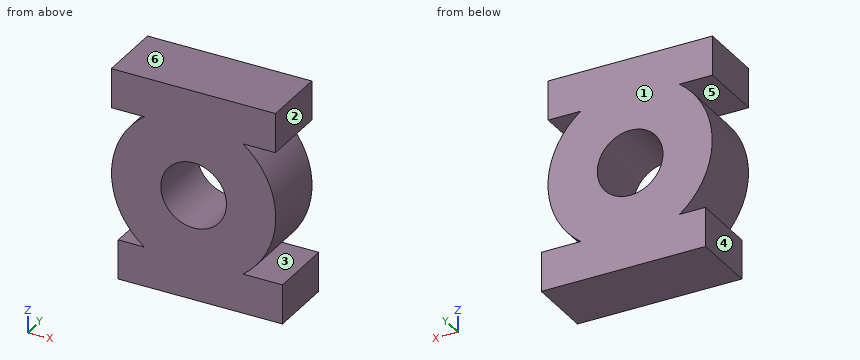
```python
from build123d import *

# Parameters (mm, degrees)
F0_R     = 12.7
F1_DEPTH = 25.4


with BuildPart() as f1:
    # F0 (on Front) → F1 (new body)
    with BuildSketch(Plane.XZ):
        with BuildLine():
            Line((-31.846212, 25.4), (-19.05, 25.4))
            ThreePointArc((-19.05, 25.4), (-31.75, 0), (-19.05, -25.4))
            Line((-19.05, -25.4), (-29.152272, -25.4))
            Line((-29.152272, -25.4), (-29.152272, -40.64))
            Line((-29.152272, -40.64), (34.347728, -40.64))
            Line((34.347728, -40.64), (34.347728, -25.4))
            Line((34.347728, -25.4), (19.05, -25.4))
            ThreePointArc((19.05, -25.4), (31.75, 0), (19.05, 25.4))
            Line((19.05, 25.4), (31.653788, 25.4))
            Line((31.653788, 25.4), (31.653788, 40.64))
            Line((31.653788, 40.64), (-31.846212, 40.64))
            Line((-31.846212, 40.64), (-31.846212, 25.4))
        make_face()
        Circle(F0_R, mode=Mode.SUBTRACT)
    extrude(amount=F1_DEPTH)


solid = f1.part
```
Model file for the job. Use its own axes, mm. Face numbers are marked on the shaded views. A direction names the side the tool comes from. Coordinates: 2 decimals unless noted, no trailing zeros. Loops run counter-clockwise (first coordinate to the right, second up) from the corner with the lowest first, then second, coordinate; pieces in that order, holes last. Notation, with made-up numbers: (-19.5, 85) -> (9.5, 85) arc R20 cw to (9.5, 107) -> close; hole circle Ø5 at (-11, 71.5). An arc over 180 degrees is marked (long way). Answer as a JSON object with one key per item and string values.
Q1. Cut at C-C (y = -17). List the corners of the cut face in (x, z), and give its area (3 significant figures).
Report:
{"outline": "(-31.85, 25.4) -> (-19.05, 25.4) arc R31.75 ccw to (-19.05, -25.4) -> (-29.15, -25.4) -> (-29.15, -40.64) -> (34.35, -40.64) -> (34.35, -25.4) -> (19.05, -25.4) arc R31.75 ccw to (19.05, 25.4) -> (31.65, 25.4) -> (31.65, 40.64) -> (-31.85, 40.64) -> close; hole circle Ø25.4 at (0, 0)", "area": "4,270 mm2"}
Q2. 3-axis set-ups, long thin cutter, end or side, ignore diameter. For the marked faces 1, 2 and 3: which of +Z, -Z, +X, -X, +Y, -Y reach the whole face in a straight line?
Report:
{"face 1": "+Z, -Z, +X, -X, +Y", "face 2": "+Z, +X, +Y, -Y", "face 3": "+X, +Y, -Y"}
Q3. Flat gauge pins, fed straight in: P1, Ø4.5, axis at y = -19, z = -32, coming from the -X side; P2, Ø8, axis at x = -4, z = 26, coming from the +Y side; P3, Ø7.5, axis at y = -7, z = 35, coming from the +X side; P4, Ø10, axis at y = -20, z = 1, coming from the -X side. Where does each tip first touch, or does it go through?
Report:
{"P1": "stops at x = -29.15", "P2": "stops at y = 0", "P3": "stops at x = 31.65", "P4": "stops at x = -31.75"}
Q4. Cut at D-D (x = 25.5). List the corners of the cut face in (y, z), and give its area (3 significant figures).
Report:
{"outline": "(-25.4, -40.64) -> (0, -40.64) -> (0, -25.4) -> (-25.4, -25.4) -> close; (-25.4, -18.92) -> (0, -18.92) -> (0, 18.92) -> (-25.4, 18.92) -> close; (-25.4, 25.4) -> (0, 25.4) -> (0, 40.64) -> (-25.4, 40.64) -> close", "area": "1,740 mm2"}
Q5. Pull direction Z, two halves, no side cores. Call the marked faces 4, 5 and 6: released by +Z, released by -Z, zero draft, split by the parting line, or undercut.
Report:
{"face 4": "zero draft", "face 5": "undercut", "face 6": "released by +Z"}
Q6. Cut at B-B (x = 0). List the corners of the cut face in (y, z).
Report:
{"outline": "(-25.4, -40.64) -> (0, -40.64) -> (0, -12.7) -> (-25.4, -12.7) -> close; (-25.4, 12.7) -> (0, 12.7) -> (0, 40.64) -> (-25.4, 40.64) -> close"}
Q7. Probe probe 1 along Z at (x, y) = (0, -17.5); probe 2 along Z at (x, y) = (-25, -8); probe 3 along Z at (x, y) = (21, -7.25). List the from-to ranges inside material, lowest first.
Report:
{"probe 1": "z = -40.64 to -12.7, 12.7 to 40.64", "probe 2": "z = -40.64 to -25.4, -19.57 to 19.57, 25.4 to 40.64", "probe 3": "z = -40.64 to -25.4, -23.81 to 23.81, 25.4 to 40.64"}
Q8. Cut at A-A (z = 0). List the corners of the cut face in (x, y), and give its area (3 significant figures).
Report:
{"outline": "(-31.75, -25.4) -> (-12.7, -25.4) -> (-12.7, 0) -> (-31.75, 0) -> close; (12.7, -25.4) -> (31.75, -25.4) -> (31.75, 0) -> (12.7, 0) -> close", "area": "968 mm2"}
